Read the model definition and answer for the solid it produces. Units are mm, in the model's axes. Face numbers are marked on the shaded views. A direction names the side the tool comes from. Coordinates: 2 decimals unless noted, no trailing zeros. Order: outer loops, then holes, each group sorted by start corner. A loop starts at its lowest first (then second) coordinate and runs counter-clockwise, first axis right, second up. Notation, with made-up numbers: M 80.5,17 L 120.5,17 A10 ccw 120.5,35 Z; hole C 78,-13.5 d10. An arc over 180 degrees is marked long. Put each result on its own line as item: value.
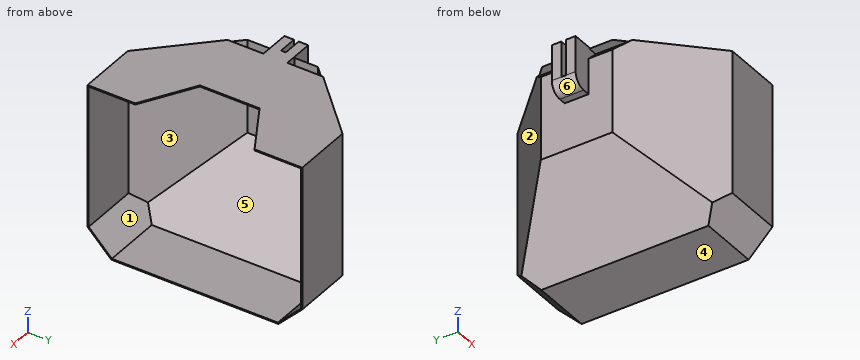
from build123d import *

# Parameters (mm, degrees)
SKETCH1_W           = 55
SKETCH1_H           = 70
BOSS_EXTRUDE1_DEPTH = 90
CHAMFER1_SIZE       = 30
CHAMFER2_SIZE       = 30
CHAMFER3_SIZE       = 10
SHELL1_T            = -0.5
SKETCH2_W           = 20
SKETCH2_H           = 5
BOSS_EXTRUDE2_DEPTH = 8
FILLET1_R           = 5
SKETCH3_W           = 30
SKETCH3_H           = 2
CUT_EXTRUDE1_DEPTH  = 8
CHAMFER5_SIZE       = 5
CUT_EXTRUDE2_DEPTH  = 5


with BuildPart() as part:
    # Sketch1 → Boss-Extrude1 (new body)
    with BuildSketch(Plane(origin=(0, 0, 0), x_dir=(1, 0, 0), z_dir=(0, 1, 0))):
        Rectangle(SKETCH1_W, SKETCH1_H)
    extrude(amount=BOSS_EXTRUDE1_DEPTH)

    # Chamfer1
    chamfer1_edges = [part.edges().sort_by_distance(p)[0] for p in [
        (-27.5, 45, -35),
    ]]
    chamfer(chamfer1_edges, length=CHAMFER1_SIZE)

    # Chamfer2
    chamfer2_edges = [part.edges().sort_by_distance(p)[0] for p in [
        (-27.5, 0, 15),
        (-27.5, 90, 15),
    ]]
    chamfer(chamfer2_edges, length=CHAMFER2_SIZE)

    # Chamfer3
    chamfer3_edges = [part.edges().sort_by_distance(p)[0] for p in [
        (15, 0, -35),
        (15, 90, -35),
    ]]
    chamfer(chamfer3_edges, length=CHAMFER3_SIZE)

    # Shell1
    shell1_openings = [part.faces().sort_by_distance(p)[0] for p in [
        (27.5, 45, 0.510752688),
    ]]
    offset(amount=SHELL1_T, openings=shell1_openings, kind=Kind.INTERSECTION)

    # Sketch2 → Boss-Extrude2 (add)
    with BuildSketch(Plane.ZY.offset(27.5)):
        with Locations((25, 47.5)):
            Rectangle(SKETCH2_W, SKETCH2_H)
        with Locations((25, 42.5)):
            Rectangle(SKETCH2_W, SKETCH2_H)
    extrude(amount=BOSS_EXTRUDE2_DEPTH)

    # Fillet1
    fillet1_edges = [part.edges().sort_by_distance(p)[0] for p in [
        (-35.5, 45, 15),
    ]]
    fillet(fillet1_edges, radius=FILLET1_R)

    # Sketch3 → Cut-Extrude1 (cut)
    with BuildSketch(Plane.ZY.offset(35.5)):
        with Locations((35, 45)):
            Rectangle(SKETCH3_W, SKETCH3_H)
    extrude(amount=-CUT_EXTRUDE1_DEPTH, mode=Mode.SUBTRACT)

    # Chamfer5
    chamfer5_edges = [part.edges().sort_by_distance(p)[0] for p in [
        (-27.5, 55, 35),
        (-27.5, 35, 35),
    ]]
    chamfer(chamfer5_edges, length=CHAMFER5_SIZE)

    # Sketch4 → Cut-Extrude2 (cut, symmetric)
    with BuildSketch(Plane(origin=(0, 0, 34.5), x_dir=(-1, 0, 0), z_dir=(0, 0, -1))):
        Polygon((-27.5, 70), (-49.150635095, 57.5), (-49.150635095, 32.5), (-27.5, 20), (-5.849364905, 32.5), (-5.849364905, 57.5), align=None)
    extrude(amount=CUT_EXTRUDE2_DEPTH, both=True, mode=Mode.SUBTRACT)


solid = part.part
Q1. Find section C-C on z = 7. Write down the section's boundary in (x, y).
Answers below:
outline: M -27.5,30 L 2.5,0 L 27.5,0 L 27.5,0.5 L 2.71,0.5 L -27,30.21 L -27,59.79 L 2.71,89.5 L 27.5,89.5 L 27.5,90 L 2.5,90 L -27.5,60 Z
Q2. A tool of negligible diameter and unlimited length cuts with its end or side. For the marked faces 5 and 6, from which of +Z, -Z, +X, -X, +Y, -Y can it reach the whole face along a straight path? Write none if from no direction.
Answers below:
face 5: +X
face 6: -Z, -X, +Y, -Y
Q3. For a pull along Z with two mould halves and no side action, classify the marked faces 1, 2, 3 and 4 as +Z half, -Z half, draft (parallel to the pull), parting line (faces both ways), or undercut.
Answers below:
face 1: undercut
face 2: draft
face 3: undercut
face 4: -Z half
Q4. Find section D-D on y = 74. Write down the section's boundary in (x, z), plus the area to 3 significant figures.
Answers below:
outline: M -13.5,-19 L 2.5,-35 L 27.5,-35 L 27.5,-34.5 L 2.71,-34.5 L -12.79,-19 L -12.79,34.5 L 27.5,34.5 L 27.5,35 L -13.5,35 Z
area: 81.9 mm^2
Q5. Find section B-B on x = 4. Write down the section's boundary in (y, z), plus the area to 3 significant figures.
Answers below:
outline: M 0,-25 L 10,-35 L 80,-35 L 90,-25 L 90,35 L 0,35 Z; hole M 0.5,-24.79 L 10.21,-34.5 L 79.79,-34.5 L 89.5,-24.79 L 89.5,34.5 L 0.5,34.5 Z
area: 153 mm^2
Q6. Given pin 1 (14.5 mm diameter, centred on x = -32, z = 20, fed in from +Y); pin 2 (1.6 mm diameter, centred on y = 45, z = 25.5, fed in from -X); pin 3 (10 mm diameter, centred on y = 52, z = -28, fed in from -X), each flat-ended and moving along its own axis, determine where each tip first touches the part or whether it passes through.
Answers below:
pin 1: stops at y = 62.75
pin 2: stops at x = -27.5
pin 3: stops at x = -9.5
Q7. Consider line 1 along Y through (x, z) = (4.5, -14); line 2 along Z through (x, y) = (17.5, 61). Determine where each line is inside the solid, lowest interval first.
Answers below:
line 1: y = 0 to 0.5, 89.5 to 90
line 2: z = -35 to -34.5
